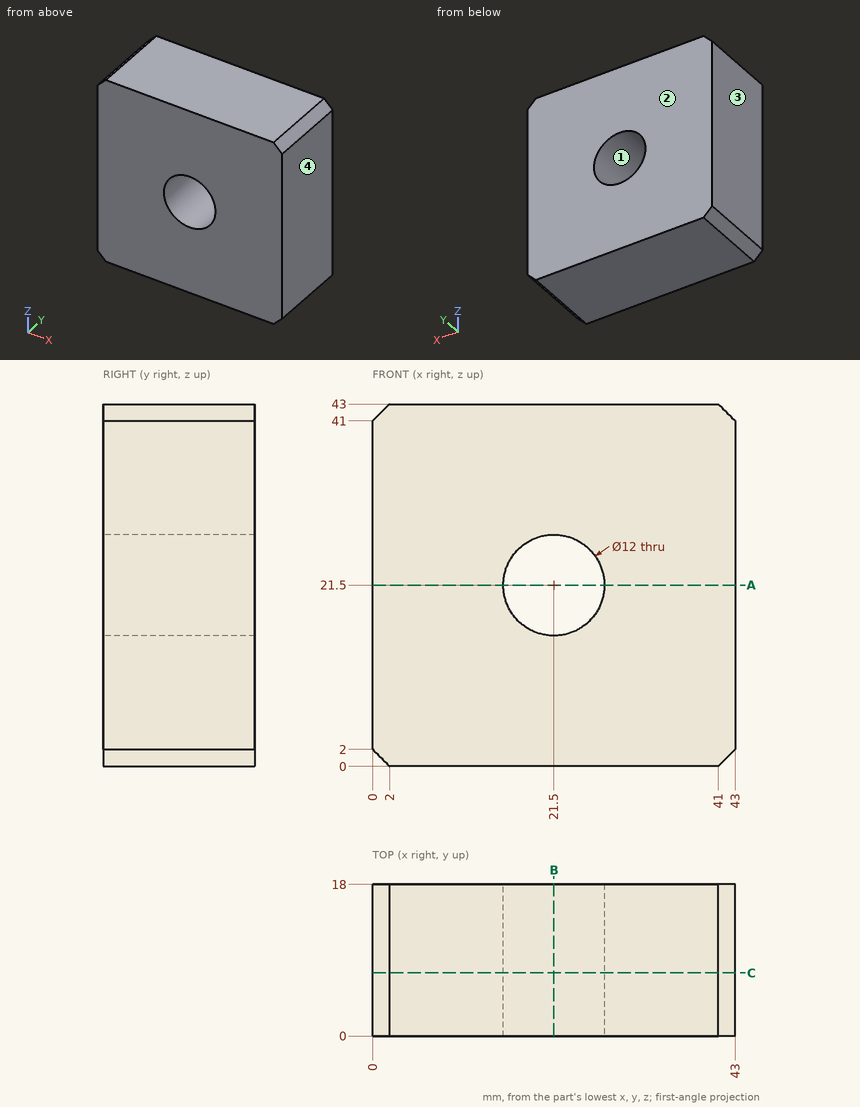
Job drawing, mm, ordinate dimensions from the low corner. One solid piece. Coordinates: 2 decimals unless noted, no trailing zeros. Write each loop counter-clockwise with the first axis right and the second up, starting at its lowest first coordinate (ties: lowest second). Pieces come first, ordered by that corner, then holes.
Item 1: Mould opens along X. For the marked faces 1, 2, 3 and 4 say: released by +X, released by -X, zero draft, split by the parting line, or undercut.
Item 2: Slice it at B-B (x = 21.5). Write the cut outline in (y, z).
Item 3: Probe line 1 (Z direction, x = 21.5, y = 13); line 2 (Z direction, x = 16.5, y = 6); line 3 (X direction, y = 12.5, z = 41.5). List the from-to ranges inside material, lowest first.
Item 4: Slice it at C-C (y = 7.5). Write the cut outline in (x, z), and give its area (3 significant figures).
Item 5: Slice it at A-A (z = 21.5). Write the cut outline in (x, y), and give its area (3 significant figures).
Item 6: Pin check, flat tip, straight feed: pin 1 (5 mm diameter, centred on y = 16, z = 19.5, fed in from -X). Stop position of the tip, or through.
Results found:
1. face 1: undercut
1. face 2: zero draft
1. face 3: released by -X
1. face 4: released by +X
2. outline: (0, 0) - (18, 0) - (18, 15.5) - (0, 15.5) - close; (0, 27.5) - (18, 27.5) - (18, 43) - (0, 43) - close
3. line 1: z = 0 to 15.5, 27.5 to 43
3. line 2: z = 0 to 18.18, 24.82 to 43
3. line 3: x = 0.5 to 42.5
4. outline: (0, 2) - (2, 0) - (41, 0) - (43, 2) - (43, 41) - (41, 43) - (2, 43) - (0, 41) - close; hole circle Ø12 at (21.5, 21.5)
4. area: 1,730 mm2
5. outline: (0, 0) - (15.5, 0) - (15.5, 18) - (0, 18) - close; (27.5, 0) - (43, 0) - (43, 18) - (27.5, 18) - close
5. area: 558 mm2
6. pin 1: stops at x = 0
